```python
from build123d import *

# Parameters (mm, degrees)
F1_DEPTH    = 7
F2_T2_ANGLE = 26.471202853
F2_T4_ANGLE = 26.471202853
F3_R        = 0.5765318272
F4_DEPTH    = 81.70182


# Not quite as in the source:
# - a fillet or chamfer that OpenCascade refuses, or shapes differently, is made with other operations: its cross-section is extruded or revolved along the edge and cut away or added


with BuildPart() as f1:
    # F0 (on Top) → F1 (new body)
    with BuildSketch(Plane.XY):
        with BuildLine():
            Line((-55.7133033872, 61.0515810549), (-59.585891664, 59.7469322383))
            ThreePointArc((-59.585891664, 59.7469322383), (-57.3715400132, 43.0123532737), (-57.6495975256, 26.1341966689))
            ThreePointArc((-57.6495975256, 26.1341966689), (-53.4588056212, 43.414181653), (-55.7133033872, 61.0515810549))
        make_face()
    extrude(amount=F1_DEPTH)

    # F2: fillet of radius 3.7881425007 on 2 edges, made by hand

    # F2_s1 → F2_t2 (revolve, cut)
    with BuildSketch(Plane(origin=(-23.8154539079, 80.2322879023, 0), x_dir=(0, 0, 1), z_dir=(-0.2845597835, 0.9586582966, 0))):
        with BuildLine():
            ThreePointArc((3.2118574993, -39.7282571763), (5.8904787496, -38.6187359259), (7, -35.9401146756))
            Line((7, -35.9401146756), (7, -39.7282571763))
            Line((7, -39.7282571763), (3.2118574993, -39.7282571763))
        make_face()
    revolve(axis=Axis((-171.3203362847, 36.4482226677, 7), (0, 0, -1)), revolution_arc=F2_T2_ANGLE, mode=Mode.SUBTRACT)

    # F2_s3 → F2_t4 (revolve, cut)
    with BuildSketch(Plane(origin=(-23.8154539079, 80.2322879023, 0), x_dir=(0, 0, 1), z_dir=(-0.2845597835, 0.9586582966, 0))):
        with BuildLine():
            ThreePointArc((3.7881425007, -39.7282571763), (1.1095212504, -38.6187359259), (0, -35.9401146756))
            Line((0, -35.9401146756), (0, -39.7282571763))
            Line((0, -39.7282571763), (3.7881425007, -39.7282571763))
        make_face()
    revolve(axis=Axis((-171.3203362847, 36.4482226677, 0), (0, 0, -1)), revolution_arc=F2_T4_ANGLE, mode=Mode.SUBTRACT)

    # F3 (on Front) → F4 (cut)
    with BuildSketch(Plane.XZ):
        with Locations((-57.4206672609, 3.7390380166)):
            Circle(F3_R)
    extrude(amount=-F4_DEPTH, mode=Mode.SUBTRACT)


solid = f1.part
```
The listing builds one solid part. Answer for the finished solid, in the listing's coordinates (mm). Round coordinates to 2 decimals unless told otherwise and drop trailing zeros. Write each loop counter-clockwise with the first axis right and the second up, starting at its lowest first coordinate (ties: lowest second). Pieces come first, ordered by that corner, then holes. Notation, with made-up numbers: (56.5, 55) -> (76.5, 55) arc R22 cw to (76.5, 80) -> close; hole circle Ø3 at (8.25, 47). An arc over 180 degrees is marked (long way). Answer as a JSON object with one key per item and string values. Group by question number.
Q1. Straight lines are drawn through the part: line 1 along X through (y, z) = (59, 1.75); line 2 along X through (y, z) = (30.5, 5.5); line 3 along Z through (x, y) = (-57.75, 55). For each, find the intervals that lie inside material, in ascending order.
Q2. Each of these flat-tipped pins is pushed along its axis until it touches: pin 1 Ø1.5 at (y, z) = (56.5, 2) entering from -X; pin 2 Ø4 at (y, z) = (51.5, 1.5) entering from +X. Where does it stop, or does it pass through?
Q3. Section B-B (z = 6) is taken. Write down the section's boundary in (x, y), plus the area to 3 significant figures.
Q4. Section A-A (z = 2) is taken. Write down the section's boundary in (x, y), plus the area to 3 significant figures.
Q5. Determine the mould class of faces 1 (the face through (-56.888, 47.052, 3.518)), 2 (the face through (-56.76, 60.7, 3.45)), 3 (the face through (-54, 52, 7)), 4 (the face through (-54, 52, 0)) for opening direction Z: pulls with the +Z half, pulls with the -Z half, needs draft (parallel to the pull), parting line crosses it, or undercut.
Check values:
{
 "1": {"line 1": "-58.83 to -55.11", "line 2": "-56.57 to -55.94", "line 3": "1.29 to 3.27, 4.21 to 5.71"},
 "2": {"pin 1": "x = -58.85", "pin 2": "x = -53.5"},
 "3": {"outline": "(-58.42, 60.14) arc R115.36 cw to (-56.14, 29.92) arc R48.98 ccw to (-55.71, 61.05) -> close", "area": "74.7 mm^2"},
 "4": {"outline": "(-59.16, 59.89) arc R114.59 cw to (-57.09, 27.44) arc R48.98 ccw to (-55.71, 61.05) -> close", "area": "99.2 mm^2"},
 "5": {"face 1": "undercut", "face 2": "needs draft", "face 3": "pulls with the +Z half", "face 4": "pulls with the -Z half"}
}
